Can you work these out from the model? Positions are in its coordinate system, mm. A direction names the side the tool comes from. Give positions to 0.01 mm unless a question says otherwise; leave off trailing zeros. Loops run counter-clockwise (first coordinate to the right, second up) from the corner with the lowest first, then second, coordinate; pieces in that order, holes last. Notation, with made-up numbers: (53.5, 10) - (85.5, 10) arc R25 cw to (85.5, 39) - close; hole circle Ø7 at (24, 7.5). An arc over 180 degrees is marked (long way). Answer as a JSON object with one key per item and string values.
```python
from build123d import *

# Parameters (mm, degrees)
SKETCH_1_R           = 5
SKETCH_1_R_2         = 2.5
EXTRUDE_1_DEPTH      = 6
SKETCH_2_R           = 2.5
EXTRUDE_2_DEPTH      = 3
SKETCH_3_R           = 1.25
CUT_EXTRUDE_3_DEPTH  = 10.273618495
EXTRUDE_START        = -12
SKETCH_8_R           = 8
SKETCH_8_R_2         = 5
EXTRUDE_4_DEPTH      = 12
SKETCH_11_R          = 1.75
CUT_EXTRUDE_4_DEPTH  = 12
SKETCH_12_R          = 1.95
CUT_EXTRUDE_5_DEPTH  = 0.5
EXTRUDE_START_2      = -10
EXTRUDE_5_DEPTH      = 10
FILLET_1_R           = 1
CUT_EXTRUDE_7_DEPTH  = 6
CUT_EXTRUDE_8_DEPTH  = 10
FILLET_2_R           = 10
EXTRUDE_START_3      = 2
EXTRUDE_6_DEPTH      = 2
EXTRUDE_7_DEPTH      = 2
CUT_EXTRUDE_9_DEPTH  = 27.588216719
EXTRUDE_START_4      = 6
SKETCH_20_R          = 5
SKETCH_20_R_2        = 3.5
EXTRUDE_8_DEPTH      = 6
SKETCH_21_R          = 1.75
CUT_EXTRUDE_10_DEPTH = 10


with BuildPart() as part:
    # 草图1 → 凸台-拉伸1 (new body)
    with BuildSketch(Plane.XY):
        Circle(SKETCH_1_R)
        Circle(SKETCH_1_R_2, mode=Mode.SUBTRACT)
    extrude(amount=EXTRUDE_1_DEPTH)

    # 草图2 → 凸台-拉伸2 (add)
    with BuildSketch(Plane.XY):
        Circle(SKETCH_2_R)
    extrude(amount=EXTRUDE_2_DEPTH)

    # 草图3 → 切除-拉伸3 (cut, through all)
    with BuildSketch(Plane.XY):
        Circle(SKETCH_3_R)
    extrude(amount=CUT_EXTRUDE_3_DEPTH, mode=Mode.SUBTRACT)

    # 草图8 → 凸台-拉伸4 (add)
    with BuildSketch(Plane.XY.offset(6).offset(EXTRUDE_START)):
        Circle(SKETCH_8_R)
        Circle(SKETCH_8_R_2, mode=Mode.SUBTRACT)
    extrude(amount=EXTRUDE_4_DEPTH)

    # 草图11 → 切除-拉伸4 (cut)
    with BuildSketch(Plane(origin=(0, 8, 0), x_dir=(1, 0, 0), z_dir=(0, 1, 0))):
        with Locations(Location((0, 3, 0), (0, 0, 270))):
            Circle(SKETCH_11_R)
    extrude(amount=-CUT_EXTRUDE_4_DEPTH, mode=Mode.SUBTRACT)

    # 草图12 → 切除-拉伸5 (cut)
    with BuildSketch(Plane(origin=(0, 8, 0), x_dir=(1, 0, 0), z_dir=(0, 1, 0))):
        with Locations(Location((0, 3, 0), (0, 0, 270))):
            Circle(SKETCH_12_R)
    extrude(amount=-CUT_EXTRUDE_5_DEPTH, mode=Mode.SUBTRACT)

    # 草图13 → 凸台-拉伸5 (add)
    with BuildSketch(Plane.XY.offset(6).offset(EXTRUDE_START_2)):
        with BuildLine():
            Line((-8, 0), (-16, 0))
            ThreePointArc((-16, 0), (0, -16), (16, 0))
            Line((16, 0), (8, 0))
            ThreePointArc((8, 0), (0, -8), (-8, 0))
        make_face()
    extrude(amount=EXTRUDE_5_DEPTH)

    # 圆角1
    fillet_1_edges = [part.edges().sort_by_distance(p)[0] for p in [
        (16, 0, 1),
        (-16, 0, 1),
    ]]
    fillet(fillet_1_edges, radius=FILLET_1_R)

    # 草图15 → 切除-拉伸7 (cut)
    with BuildSketch(Plane(origin=(0, 0, -4), x_dir=(-1, 0, 0), z_dir=(0, 0, -1))):
        with BuildLine():
            Line((-10, 0), (-8, 0))
            ThreePointArc((-8, 0), (0, -8), (8, 0))
            Line((8, 0), (10, 0))
            ThreePointArc((10, 0), (0, -10), (-10, 0))
        make_face()
    extrude(amount=-CUT_EXTRUDE_7_DEPTH, mode=Mode.SUBTRACT)

    # 草图16 → 切除-拉伸8 (cut)
    with BuildSketch(Plane(origin=(0, 0, -4), x_dir=(-1, 0, 0), z_dir=(0, 0, -1))):
        with BuildLine():
            Line((11.661330827, 0), (14.966629547, 0))
            ThreePointArc((14.966629547, 0), (15.69692629, -0.316869949), (15.96440485, -1.066666667))
            ThreePointArc((15.96440485, -1.066666667), (13.334766709, -8.842171499), (7.195716327, -14.290614631))
            ThreePointArc((7.195716327, -14.290614631), (10.518928308, -7.486043338), (11.661330827, 0))
        make_face()
    extrude(amount=-CUT_EXTRUDE_8_DEPTH, mode=Mode.SUBTRACT)

    # 圆角2
    fillet_2_edges = [part.edges().sort_by_distance(p)[0] for p in [
        (-7.195716327, -14.290614631, 1),
    ]]
    fillet(fillet_2_edges, radius=FILLET_2_R)

    # 草图17 → 凸台-拉伸6 (add)
    with BuildSketch(Plane(origin=(0, 0, -4), x_dir=(-1, 0, 0), z_dir=(0, 0, -1)).offset(EXTRUDE_START_3)):
        with BuildLine():
            Line((10, 0), (11.661330827, 0))
            ThreePointArc((11.661330827, 0), (11.141957729, -5.079523953), (9.605333334, -9.948825493))
            ThreePointArc((9.605333334, -9.948825493), (6.210515001, -14.141064577), (1.131984253, -15.95990638))
            ThreePointArc((1.131984253, -15.95990638), (-10.509629988, -12.064314217), (-15.96440485, -1.066666667))
            ThreePointArc((-15.96440485, -1.066666667), (-15.69692629, -0.316869949), (-14.966629547, 0))
            Line((-14.966629547, 0), (-10, 0))
            ThreePointArc((-10, 0), (0, -10), (10, 0))
        make_face()
    extrude(amount=-EXTRUDE_6_DEPTH)

    # 草图18 → 凸台-拉伸7 (add)
    with BuildSketch(Plane(origin=(0, 0, -6), x_dir=(-1, 0, 0), z_dir=(0, 0, -1)).offset(EXTRUDE_START_3)):
        with BuildLine():
            Line((10, 0), (11.661330827, 0))
            ThreePointArc((11.661330827, 0), (11.141957729, -5.079523953), (9.605333334, -9.948825493))
            ThreePointArc((9.605333334, -9.948825493), (6.210515001, -14.141064577), (1.131984253, -15.95990638))
            ThreePointArc((1.131984253, -15.95990638), (-10.509629988, -12.064314217), (-15.96440485, -1.066666667))
            ThreePointArc((-15.96440485, -1.066666667), (-15.69692629, -0.316869949), (-14.966629547, 0))
            Line((-14.966629547, 0), (-10, 0))
            Line((-10, 0), (-8, 0))
            Line((-8, 0), (-5, 0))
            ThreePointArc((-5, 0), (0, -5), (5, 0))
            Line((5, 0), (8, 0))
            Line((8, 0), (10, 0))
        make_face()
    extrude(amount=-EXTRUDE_7_DEPTH)

    # 草图19 → 切除-拉伸9 (cut, through all)
    with BuildSketch(Plane(origin=(0, 0, -8), x_dir=(-1, 0, 0), z_dir=(0, 0, -1))):
        with BuildLine():
            Line((11.661330827, 0), (11.5, 0))
            ThreePointArc((11.5, 0), (0, -11.5), (-11.5, 0))
            Line((-11.5, 0), (-14.966629547, 0))
            ThreePointArc((-14.966629547, 0), (-15.69692629, -0.316869949), (-15.96440485, -1.066666667))
            ThreePointArc((-15.96440485, -1.066666667), (-10.509629988, -12.064314217), (1.131984253, -15.95990638))
            ThreePointArc((1.131984253, -15.95990638), (6.210515001, -14.141064577), (9.605333334, -9.948825493))
            ThreePointArc((9.605333334, -9.948825493), (11.141957729, -5.079523953), (11.661330827, 0))
        make_face()
    extrude(amount=-CUT_EXTRUDE_9_DEPTH, mode=Mode.SUBTRACT)

    # 草图20 → 凸台-拉伸8 (add)
    with BuildSketch(Plane(origin=(0, 0, 0), x_dir=(-1, 0, 0), z_dir=(0, 0, -1)).offset(EXTRUDE_START_4)):
        Circle(SKETCH_20_R)
        with Locations(Location((0, 0, 0), (0, 0, 180))):
            Circle(SKETCH_20_R_2, mode=Mode.SUBTRACT)
    extrude(amount=-EXTRUDE_8_DEPTH)

    # 草图21 → 切除-拉伸10 (cut)
    with BuildSketch(Plane(origin=(0, 8, 0), x_dir=(1, 0, 0), z_dir=(0, 1, 0))):
        with Locations(Location((0, 3, 0), (0, 0, 270))):
            Circle(SKETCH_21_R)
    extrude(amount=-CUT_EXTRUDE_10_DEPTH, mode=Mode.SUBTRACT)


solid = part.part
```
1) I need wall thicknesses on L1, parallel to Y at x = 0, z = 1.3; L2, parallel to Z at x = -9.25, y = -2.5; L3, parallel to X at y = -4.75, z = -2.75. Which ranges of each line are inside material? Lowest first, please.
Check sheet entries:
{"L1": "-11.5 to -10, -8 to -1.25, 1.25 to 8", "L2": "-8 to -6, 2 to 6", "L3": "-10.47 to -8.8, -6.44 to 6.44, 8.8 to 10.47"}
2) Imagine slicing it at C-C on z = -3. Write out the boundary of the cut face in (x, y), and give its area (3 significant figures).
Check sheet entries:
{"outline": "(-11.5, 0) arc R11.5 ccw to (11.5, 0) - (10, 0) arc R10 cw to (-10, 0) - close; (-1.95, 7.5) - (-1.95, 7.76) arc R8 ccw (long way) to (1.95, 7.76) - (1.95, 7.5) - (1.75, 7.5) - (1.75, 3.03) arc R3.5 cw (long way) to (-1.75, 3.03) - (-1.75, 7.5) - close", "area": "197 mm2"}
3) Which directions (+Z, -Z, +X, -X, +Y, -Y) give clear straight access to the entire face, cutting with the end or side of a thin tool? Please do faces 1 (the flat face through (0, -8.3, 2)), 2 (the cylindrical face through (-0.54, -2.44, 4.48)), 3 (the cylindrical face through (0, -5, -7)).
Check sheet entries:
{"face 1": "none", "face 2": "+Z", "face 3": "-Z, +Y"}
4) I'm going to push flat-ended pins straight in: P1, Ø6, axis at y = 6, z = 2, coming from the -X side; P2, Ø8, axis at x = 9, z = -5, coming from the -Y side; P3, Ø6, axis at x = 7.5, y = 5.5, coming from the -Z side; P4, Ø2, axis at x = 0, y = 0, coming from the +Z side (3 decimals). Where does each tip first touch, or does it pass through?
Check sheet entries:
{"P1": "x = -7.42", "P2": "y = -10.36", "P3": "z = -6", "P4": "through"}
5) If we mould it in two halves opening along Y, with no side actions, what happens to faces 4 (the flat face through (10.5, 0, -1.1)), 5 (the cylindrical face through (-0.253, -11.497, -1.098)), 6 (the flat face through (0, 4, -6)), 7 (the flat face through (-1, -1, 3))? For each: released by +Y, released by -Y, zero draft, split by the parting line, or undercut.
Check sheet entries:
{"face 4": "released by +Y", "face 5": "released by -Y", "face 6": "zero draft", "face 7": "undercut"}
6) Imagine slicing it at A-A on x = 0. Give the number of separate pieces and of enclosed holes in the cut face, and give its area (3 significant figures).
Check sheet entries:
{"separate pieces": "3", "enclosed holes": "1", "area": "151 mm2"}
7) Imagine slicing it at D-D on y = -8.5. Write out the boundary of the cut face in (x, z), and give its area (3 significant figures).
Check sheet entries:
{"outline": "(-7.75, -8) - (7.75, -8) - (7.75, 6) - (-7.75, 6) - close; hole (-5.27, -6) - (5.27, -6) - (5.27, 2) - (-5.27, 2) - close", "area": "133 mm2"}
8) Imagine slicing it at B-B on z = 1.5. Write out the boundary of the cut face in (x, y), and give its area (3 significant figures).
Check sheet entries:
{"outline": "(-11.5, 0) arc R11.5 ccw to (11.5, 0) - (10, 0) arc R10 cw to (-10, 0) - close; circle Ø16 at (0, 0); hole circle Ø2.5 at (0, 0)", "area": "247 mm2"}
